Verification items for the finished model (mm, model axes). A direction names the side the tool comes from. Give positions to 0.01 mm unless a question says otherwise; leave off trailing zeros. Order: outer loops, then holes, each group sorted by start corner. A loop starts at its lowest first (then second) coordinate and runs counter-clockwise, first axis right, second up. Notation, with made-up numbers: (52.25, -12.75) - (74.25, -12.75) arc R22 ccw to (74.25, -5.75) - close; hole circle Ø6 at (17.25, -3.5). An arc over 180 degrees is marked (long way). Answer as a JSON object with one key per item and string values.
```python
from build123d import *

# Parameters (mm, degrees)
EXTRUDE_1_DEPTH     = 13
CUT_EXTRUDE_1_DEPTH = 49.114446895


with BuildPart() as part:
    # 草图1 → 凸台-拉伸1 (new body)
    with BuildSketch(Plane(origin=(0, 0, 0), x_dir=(1, 0, 0), z_dir=(0, 1, 0))):
        with BuildLine():
            Line((20, 0), (25, 0))
            ThreePointArc((25, 0), (21.416586692, 18), (25, 36))
            Line((25, 36), (25, 39))
            Line((25, 39), (22, 39))
            ThreePointArc((22, 39), (5.87927664, 22.388613177), (0, 0))
            Line((0, 0), (0, -6))
            Line((0, -6), (20, -6))
            Line((20, -6), (20, 0))
        make_face()
        with BuildLine():
            ThreePointArc((16.080059058, 29.907367254), (8.618420181, 19.967852036), (4.392399403, 8.279791209))
            ThreePointArc((4.392399403, 8.279791209), (4.947419472, 6.462870357), (6.770848151, 5.929619467))
            ThreePointArc((6.770848151, 5.929619467), (11.882919882, 6.480681597), (16.999608279, 5.974275931))
            ThreePointArc((16.999608279, 5.974275931), (18.809570487, 6.514692506), (19.362380146, 8.320908094))
            ThreePointArc((19.362380146, 8.320908094), (18.417004852, 18.204489029), (19.4431912, 28.080006643))
            ThreePointArc((19.4431912, 28.080006643), (18.439109127, 30.240549881), (16.080059058, 29.907367254))
        make_face(mode=Mode.SUBTRACT)
    extrude(amount=EXTRUDE_1_DEPTH)

    # 草图2 → 切除-拉伸1 (cut, through all)
    with BuildSketch(Plane.ZY):
        Polygon((1.746538635, 13), (1.746538635, 9.75), (6, 10.5), (6, 13), align=None)
        Polygon((6, 2.5), (6, 0), (1.746538635, 0), (1.746538635, 3.25), align=None)
    extrude(amount=-CUT_EXTRUDE_1_DEPTH, mode=Mode.SUBTRACT)


solid = part.part
```
(1) Section check C-C (y = 6.75). Record the cut outline in (x, z).
Computed values:
{"outline": "(0, 0) arc R45.57 ccw to (22, -39) - (25, -39) - (25, -36) arc R47 cw to (25, 0) - (20, 0) - (20, 6) - (0, 6) - close; hole (4.39, -8.28) arc R42 ccw to (16.08, -29.91) arc R2 ccw to (19.44, -28.08) arc R50 cw to (19.36, -8.32) arc R2 ccw to (17, -5.97) arc R25 cw to (6.77, -5.93) arc R2 ccw to start"}
(2) Material ranges on line 1 along Z through (x, y) = (9.75, 12.5); line 2 along Z through (x, y) = (7, 4); line 3 along X through (y, z) = (2, -22), recorded low to high. Write a range as [from, to].
Computed values:
{"line 1": "z = [-28.17, -21.93], [-6.38, 1.75]", "line 2": "z = [-24.27, -16.63], [-5.98, 6]", "line 3": "x = [5.66, 9.79], [18.58, 21.59]"}
(3) Section check D-D (x = 5.75). Record the cut outline in (y, z), then the cut area to 3 significant figures.
Computed values:
{"outline": "(0, -22.16) - (13, -22.16) - (13, -13.36) - (0, -13.36) - close; (0, -5.98) - (13, -5.98) - (13, 1.75) - (9.75, 1.75) - (10.5, 6) - (2.5, 6) - (3.25, 1.75) - (0, 1.75) - close", "area": "246 mm²"}
(4) Section check B-B (z = -25). Record the cut outline in (x, y).
Computed values:
{"outline": "(7.47, 0) - (11.82, 0) - (11.82, 13) - (7.47, 13) - close; (18.91, 0) - (21.94, 0) - (21.94, 13) - (18.91, 13) - close"}
(5) Access from +Z, -Z, +X, -X, +Y, -Y to the whole of each face (thin tool, end or side, straight path). Record for faces 4 (the flat face through (10, 2, 1.747)), 5 (the flat face through (10, 11, 1.747)), 6 (the cylindrical face through (11.81, 6.41, -6.48)).
Computed values:
{"face 4": "+X, -X, -Y", "face 5": "+X, -X, +Y", "face 6": "+Y, -Y"}
(6) Gauge pin test, flat ends, axial feed: pin 1 Ø2 at (y, z) = (3.5, -4.5) entering from +X; pin 2 Ø2.5 at (x, y) = (23.5, 4) entering from +Z; pin 3 Ø3 at (y, z) = (4.5, -29.5) entering from -X. Record the tip position at first contact, or that the pin passes through.
Computed values:
{"pin 1": "stops at x = 23.71", "pin 2": "stops at z = 0", "pin 3": "stops at x = 9.62"}
(7) Release check for a two-part mould opening along Z. For faces 1 (the flat face through (24, 6, -39)), 2 (the flat face through (9.86, 2.88, 3.84)), 3 (the flat face through (22, 6, 0)) record: pulls with the +Z half, pulls with the -Z half, needs draft (parallel to the pull), parting line crosses it, or undercut.
Computed values:
{"face 1": "pulls with the -Z half", "face 2": "undercut", "face 3": "pulls with the +Z half"}
(8) Section check A-A (x = 9.5). Record the cut outline in (y, z), then the cut area to 3 significant figures.
Computed values:
{"outline": "(0, -27.85) - (13, -27.85) - (13, -21.52) - (0, -21.52) - close; (0, -6.36) - (13, -6.36) - (13, 1.75) - (9.75, 1.75) - (10.5, 6) - (2.5, 6) - (3.25, 1.75) - (0, 1.75) - close", "area": "218 mm²"}
